from build123d import *

# Parameters (mm, degrees)
F0_W        = 75
F0_H        = 120
F1_DEPTH    = 10
F2_R        = 1.5
F3_DEPTH    = 41.3
F4_W        = 75
F4_H        = 59.0305535599
F5_DEPTH    = 40
F7_R        = 10
F6_W        = 12.5
F6_H        = 59.0305535599
F6_W_2      = 10
F8_DEPTH    = 40
F9_T1_DEPTH = 160
F9_T3_DEPTH = 160
F9_T5_DEPTH = 160
F10_R       = 1.5
F11_DEPTH   = 57.1


# Not quite as in the source:
# - a fillet or chamfer that OpenCascade refuses, or shapes differently, is made with other operations: its cross-section is extruded or revolved along the edge and cut away or added


with BuildPart() as f1:
    # F0 (on Front) → F1 (new body)
    with BuildSketch(Plane.XZ):
        Rectangle(F0_W, F0_H)
    extrude(amount=F1_DEPTH)

    # F2 (on face) → F3 (cut)
    with BuildSketch(Plane.XZ.offset(10)):
        with Locations((0, -45)):
            Circle(F2_R)
        with Locations((0, 45)):
            Circle(F2_R)
    extrude(amount=-F3_DEPTH, mode=Mode.SUBTRACT)

    # F4 (on face) → F5 (join)
    with BuildSketch(Plane.XZ.offset(10)):
        Rectangle(F4_W, F4_H)
    extrude(amount=F5_DEPTH)

    # F7
    f7_edges = [f1.edges().sort_by_distance(p)[0] for p in [
        (37.5, -5, 60),
        (-37.5, -5, 60),
        (-37.5, -5, -60),
        (37.5, -5, -60),
    ]]
    fillet(f7_edges, radius=F7_R)

    # F6 (on face) → F8 (cut)
    with BuildSketch(Plane.XZ.offset(50)):
        with Locations((-31.25, 0)):
            Rectangle(F6_W, F6_H)
        with Locations((-10, 0)):
            Rectangle(F6_W_2, F6_H)
        with Locations((10, 0)):
            Rectangle(F6_W_2, F6_H)
        with Locations((31.25, 0)):
            Rectangle(F6_W, F6_H)
    extrude(amount=-F8_DEPTH, mode=Mode.SUBTRACT)

    # F9: fillet of radius 30 on 6 edges, made by hand

    # F9_s2 → F9_t1 (cut)
    with BuildSketch(Plane.YZ.offset(-60)):
        with BuildLine():
            ThreePointArc((-50, -0.4847232201), (-41.2132034356, 20.7284802155), (-20, 29.5152767799))
            Line((-20, 29.5152767799), (-50, 29.5152767799))
            Line((-50, 29.5152767799), (-50, -0.4847232201))
        make_face()
        with BuildLine():
            ThreePointArc((-50, 0.4847232201), (-41.2132034356, -20.7284802155), (-20, -29.5152767799))
            Line((-20, -29.5152767799), (-50, -29.5152767799))
            Line((-50, -29.5152767799), (-50, 0.4847232201))
        make_face()
    extrude(amount=F9_T1_DEPTH, mode=Mode.SUBTRACT)

    # F9_s4 → F9_t3 (cut)
    with BuildSketch(Plane.YZ.offset(-80)):
        with BuildLine():
            ThreePointArc((-50, -0.4847232201), (-41.2132034356, 20.7284802155), (-20, 29.5152767799))
            Line((-20, 29.5152767799), (-50, 29.5152767799))
            Line((-50, 29.5152767799), (-50, -0.4847232201))
        make_face()
        with BuildLine():
            ThreePointArc((-50, 0.4847232201), (-41.2132034356, -20.7284802155), (-20, -29.5152767799))
            Line((-20, -29.5152767799), (-50, -29.5152767799))
            Line((-50, -29.5152767799), (-50, 0.4847232201))
        make_face()
    extrude(amount=F9_T3_DEPTH, mode=Mode.SUBTRACT)

    # F9_s6 → F9_t5 (cut)
    with BuildSketch(Plane.YZ.offset(-100)):
        with BuildLine():
            ThreePointArc((-50, -0.4847232201), (-41.2132034356, 20.7284802155), (-20, 29.5152767799))
            Line((-20, 29.5152767799), (-50, 29.5152767799))
            Line((-50, 29.5152767799), (-50, -0.4847232201))
        make_face()
        with BuildLine():
            ThreePointArc((-50, 0.4847232201), (-41.2132034356, -20.7284802155), (-20, -29.5152767799))
            Line((-20, -29.5152767799), (-50, -29.5152767799))
            Line((-50, -29.5152767799), (-50, 0.4847232201))
        make_face()
    extrude(amount=F9_T5_DEPTH, mode=Mode.SUBTRACT)

    # F10 (on face) → F11 (cut)
    with BuildSketch(Plane.YZ.offset(25)):
        with Locations((-39.9960838011, 0)):
            Circle(F10_R)
    extrude(amount=-F11_DEPTH, mode=Mode.SUBTRACT)


solid = f1.part
Source: CAD feature listing. Evaluate the final solid. Frame: model axes, mm. A direction names the side the tool comes from. Round coordinates to 2 decimals unless told otherwise and drop trailing zeros. Loops run counter-clockwise (first coordinate to the right, second up) from the corner with the lowest first, then second, coordinate; pieces in that order, holes last. Notation, with made-up numbers: (37.5, -3.75) -> (94.5, -3.75) arc R17 ccw to (94.5, 3.25) -> close; hole circle Ø11 at (71.5, 81.25). An arc over 180 degrees is marked (long way). Answer as a JSON object with one key per item and string values. Group by question number.
Q1. Section query D-D (z = 19.5). Output: boundary loops of the cut face in (x, y), plus the area to 3 significant figures.
Q2. Access query for faces 5 (the flat face through (0, -15, -29.515)), 6 (the flat face through (-25, -26, 0)), 7 (the flat face through (25, -26, 0)), 8 (the flat face through (-20, -15, 29.515)). Directions: +Z, -Z, +X, -X, +Y, -Y. A direction counts if a zero-diameter tool reaches every point of the face in a straight line with its end or side. Return the directions, or none.
Q3. Section query A-A (x = 0). Output: boundary loops of the cut face in (y, z).
Q4. Section query C-C (y = -12). Output: boundary loops of the cut face in (x, z), plus the area to 3 significant figures.
Q5. Section query B-B (z = -45). Output: boundary loops of the cut face in (x, y).
Q6. Contact query for flat-ended pins moving along their axis: P1, Ø3, axis at x = -22.5, y = -15.5, coming from the +Z side; P2, Ø3, axis at y = -32.5, z = 11, coming from the +X side; P3, Ø12, axis at y = -36.5, z = -7, coming from the -X side. Output: stop coordinate, or through.
Q7. Mould query, pull axis Z, two halves, no side actions, for faces 1 (the cylindrical face through (-19.93, -38.565, 0.451)), 2 (the flat face through (15, -26, 0)), 3 (the cylindrical face through (-34.65, -5.07, -56.99)), 4 (the cylindrical face through (0.07, -38.565, 0.451)). Classes: pulls with the +Z half, pulls with the -Z half, needs draft (parallel to the pull), parting line crosses it, or undercut.
Q8. Ray query, line 1 (X direction, y = -28.5, z = 13.5); line 2 (Z direction, x = 0, y = -3); line 3 (Y direction, x = 27, z = 24). Return the intervals inside material, ascending. Write a range as from..to.
Completed:
{
 "1": {"outline": "(-37.5, -10) -> (-25, -10) -> (-25, -42.37) -> (-15, -42.37) -> (-15, -10) -> (-5, -10) -> (-5, -42.37) -> (5, -42.37) -> (5, -10) -> (15, -10) -> (15, -42.37) -> (25, -42.37) -> (25, -10) -> (37.5, -10) -> (37.5, 0) -> (-37.5, 0) -> close", "area": "1,720 mm²"},
 "2": {"face 5": "-Z, +X, -X, -Y", "face 6": "+Z, -Z, -X, -Y", "face 7": "+Z, -Z, +X, -Y", "face 8": "+Z, +X, -X, -Y"},
 "3": {"outline": "(-50, 0) arc R30 ccw to (-20, -29.52) -> (-10, -29.52) -> (-10, -43.5) -> (0, -43.5) -> (0, 43.5) -> (-10, 43.5) -> (-10, 29.52) -> (-20, 29.52) arc R30 ccw to start; (-10, -60) -> (0, -60) -> (0, -46.5) -> (-10, -46.5) -> close; (-10, 46.5) -> (0, 46.5) -> (0, 60) -> (-10, 60) -> close; hole circle Ø3 at (-40, 0)"},
 "4": {"outline": "(-25, -29.52) -> (-15, -29.52) -> (-15, 29.52) -> (-25, 29.52) -> close; (-5, -29.52) -> (5, -29.52) -> (5, 29.52) -> (-5, 29.52) -> close; (15, -29.52) -> (25, -29.52) -> (25, 29.52) -> (15, 29.52) -> close", "area": "1,770 mm²"},
 "5": {"outline": "(-37.5, -10) -> (-1.5, -10) -> (-1.5, 0) -> (-37.5, 0) -> close; (1.5, -10) -> (37.5, -10) -> (37.5, 0) -> (1.5, 0) -> close"},
 "6": {"P1": "z = 29.52", "P2": "x = 25", "P3": "x = -25"},
 "7": {"face 1": "undercut", "face 2": "needs draft", "face 3": "pulls with the -Z half", "face 4": "undercut"},
 "8": {"line 1": "-25..-15, -5..5, 15..25", "line 2": "-60..-46.5, -43.5..43.5, 46.5..60", "line 3": "-10..0"}
}
